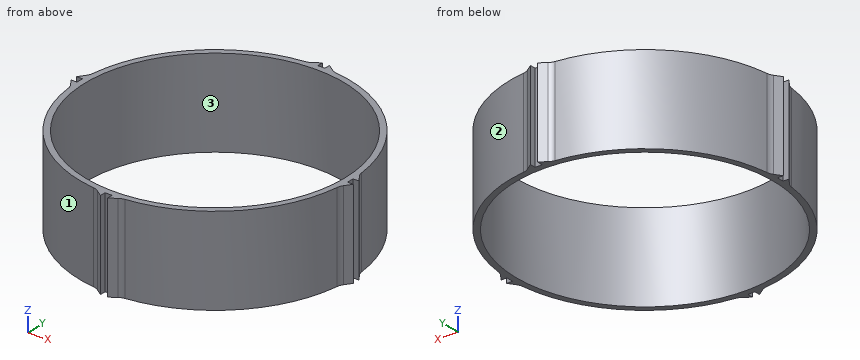
Autodesk Inventor part; units mm, degrees
ref_plane "YZ Plane" through (0, 0, 0) normal (1, 0, 0) x (0, 1, 0)
ref_plane "XZ Plane" through (0, 0, 0) normal (0, 1, 0) x (-1, 0, 0)
ref_plane "XY Plane" through (0, 0, 0) normal (0, 0, 1) x (1, 0, 0)
sketch "Sketch1" plane through (0, 0, 0) normal (0, 0, 1) x (1, 0, 0)
  circle A0 centre (0, 0) radius 14.605
  circle A1 centre (0, 0) radius 13.97
  dimension "d0" = 29.21
  dimension "d1" = 27.94
extrude "Extrusion1" add sketch "Sketch1" along normal blind 9.525
sketch "Sketch2" plane through (0, 0, 9.525) normal (0, 0, 1) x (1, 0, 0)
  circle A0 centre (0, 0) radius 13.97
  circle A1 centre (0, 0) radius 14.605
  line L0 (0.381, 14.6) -> (-0.381, 14.6)
  line L1 (0.381, 14.6) -> (0.381, 15.235)
  line L2 (0.381, 15.235) -> (-0.381, 15.235)
  line L3 (-0.381, 15.235) -> (-0.381, 14.6)
  line L4 (-0.381, 15.235) -> (-1.3732, 14.5403)
  line L5 (-0.381, 15.235) -> (0.8302, 15.235) construction
  circle A2 centre (0, 0) radius 14.605
  line L6 (0.381, 15.235) -> (1.3732, 14.5403)
  line L7 (0.381, 15.235) -> (1.5922, 15.235) construction
  dimension "d4" = 0.762
  dimension "d5" = 0.635
  dimension "d8" = 145
  dimension "d9" = 35
extrude "Extrusion2" add sketch "Sketch2" against normal blind 9.525 contours A1 L1 L6 | L4 L3 A1 | L0 A1 picked at (0.0423, 14.6015)
fillet "Fillet1" radius 1.27 2 edges at (1.3732, 14.5403, 4.7625) (-1.3732, 14.5403, 4.7625)
extrude "Extrusion3" cut sketch "Sketch2" against normal blind 9.525 contours L0 A1 picked at (0.0423, 14.6015)
pattern_circular "Circular Pattern2" count 4 over 360 about axis through (0, 0, 0) along (0, 0, 1) of "Extrusion3", "Extrusion2", "Fillet1"
properties part number "PropShroud"
Check sheet for the modelled part. Datum: model origin and axes. Units: mm. Face numbers are marked on the shaded views. Round coordinates to 2 decimals unless told otherwise and drop trailing zeros. Order: outer loops, then holes, each group sorted by start corner. A loop starts at its lowest first (then second) coordinate and runs counter-clockwise, first axis right, second up.
(1) Scan lines: probe 1 along Y at (x, z) = (0, 7) (3 decimals); probe 2 along X at (y, z) = (-1.5, 7.25); probe 3 along X at (y, z) = (12.5, 8.75). Record each from-to range of solid material in increasing order.
(2) Cross-section at B-B, the plane y = 0. Enter the section's corners in (x, z) (3 decimals).
(3) Draft check along Y on the marked faces 1, 2 and 3. Enter one of: pulls with the +Y half, pulls with the -Y half, needs draft (parallel to the pull), parting line crosses it, or undercut.
(4) Cross-section at A-A, the plane x = 0. Enter the section's corners in (y, z) (3 decimals).
(5) Go/stop test with flat-tipped pins: P1, Ø0.5, axis at x = -15, z = 3, coming from the +Y side; P2, Ø0.5, axis at y = 15, z = 5, coming from the -X side; P3, Ø0.5, axis at x = -15, z = 2.5, coming from the -Y side. Record where each tip stops, or that it passes through.
Check sheet entries:
1. probe 1: y = -14.605 to -13.97, 13.97 to 14.6
1. probe 2: x = -14.54 to -13.89, 13.89 to 14.54
1. probe 3: x = -7.55 to -6.24, 6.24 to 7.55
2. outline: (-14.605, 0) - (-13.97, 0) - (-13.97, 9.525) - (-14.605, 9.525) - close; (13.97, 0) - (14.605, 0) - (14.605, 9.525) - (13.97, 9.525) - close
3. face 1: pulls with the -Y half
3. face 2: pulls with the +Y half
3. face 3: undercut
4. outline: (-14.605, 0) - (-13.97, 0) - (-13.97, 9.525) - (-14.605, 9.525) - close; (13.97, 0) - (14.6, 0) - (14.6, 9.525) - (13.97, 9.525) - close
5. P1: stops at y = 1.07
5. P2: stops at x = -1.07
5. P3: stops at y = -1.07
